from build123d import *

# Parameters (mm, degrees)
BASE_FLANGE1_DEPTH = 20
SKETCH6_R          = 2
CUT_EXTRUDE1_DEPTH = 10
SKETCH7_R          = 2
CUT_EXTRUDE2_DEPTH = 3


# Sheet-metal steps are written as plain solids
with BuildPart() as part:
    # Sketch1 → Base-Flange1 (new body)
    with BuildSketch(Plane(origin=(0, 0, 0), x_dir=(0, 0, -1), z_dir=(1, 0, 0))):
        with BuildLine():
            Line((0, 20), (0, 2))
            ThreePointArc((0, 2), (-0.585786438, 0.585786438), (-2, 0))
            Line((-2, 0), (-20, 0))
            Line((-20, 0), (-20, -3))
            Line((-20, -3), (-2, -3))
            ThreePointArc((-2, -3), (1.535533906, -1.535533906), (3, 2))
            Line((3, 2), (3, 20))
            Line((3, 20), (0, 20))
        make_face()
    extrude(amount=BASE_FLANGE1_DEPTH)

    # Sketch6 → Cut-Extrude1 (cut)
    with BuildSketch(Plane(origin=(0, 0, -3), x_dir=(-1, 0, 0), z_dir=(0, 0, -1))):
        with Locations(Location((-10, 11, 0), (0, 0, 90))):
            Circle(SKETCH6_R)
    extrude(amount=-CUT_EXTRUDE1_DEPTH, mode=Mode.SUBTRACT)

    # Sketch7 → Cut-Extrude2 (cut)
    with BuildSketch(Plane.XZ.offset(3)):
        with Locations(Location((10, 11, 0), (0, 0, 270))):
            Circle(SKETCH7_R)
    extrude(amount=-CUT_EXTRUDE2_DEPTH, mode=Mode.SUBTRACT)


solid = part.part
CAD build for the part. Positions are in the model's coordinates, mm. A direction names the side the tool comes from. Round coordinates to 2 decimals unless told otherwise and drop trailing zeros. Order: outer loops, then holes, each group sorted by start corner. A loop starts at its lowest first (then second) coordinate and runs counter-clockwise, first axis right, second up. Notation, with made-up numbers: (-22, 27) -> (9, 27) arc R18 cw to (9, 53) -> close; hole circle Ø7 at (26, 25.25). An arc over 180 degrees is marked (long way). Write each question's results on one line, items separated by ' | '.
1. Wall check: line 1 along X through (y, z) = (-1.35, 11); line 2 along Z through (x, y) = (10, 16). Give the ranges that are in metal, low to high. Write a range as [from, to].
Findings below:
line 1: x = [0, 8], [12, 20] | line 2: z = [-3, 0]
2. Flat gauge pins, fed straight in: P1, Ø5, axis at x = 10, z = 11, coming from the +Y side; P2, Ø5, axis at x = 10, y = 11, coming from the +Z side; P3, Ø1.5, axis at y = 2, z = 6, coming from the +X side. Where does each tip first touch, or does it go through?
Findings below:
P1: stops at y = 0 | P2: stops at z = 0 | P3: passes through
3. Pull direction Y, two halves, no side cores. Call faces 1 (the face through (0, -1, 4)), 2 (the face through (11.352, 9.526, -1.521)), 3 (the face through (7.6, 0, 10.9)): pulls with the +Y half, pulls with the -Y half, needs draft (parallel to the pull), parting line crosses it, or undercut.
Findings below:
face 1: needs draft | face 2: undercut | face 3: pulls with the +Y half
4. Cut at B-B (x = 10). Give the cut face in (y, z).
Findings below:
outline: (-3, 2) arc R5 ccw to (2, -3) -> (9, -3) -> (9, 0) -> (2, 0) arc R2 cw to (0, 2) -> (0, 9) -> (-3, 9) -> close; (-3, 13) -> (0, 13) -> (0, 20) -> (-3, 20) -> close; (13, -3) -> (20, -3) -> (20, 0) -> (13, 0) -> close
5. Cut at D-D (x = 4.5). Give the cut face in (y, z), plus the area to 3 significant figures.
Findings below:
outline: (-3, 2) arc R5 ccw to (2, -3) -> (20, -3) -> (20, 0) -> (2, 0) arc R2 cw to (0, 2) -> (0, 20) -> (-3, 20) -> close | area: 124 mm²
6. Cut at A-A (z = 11). Give the cut face in (x, y).
Findings below:
outline: (0, -3) -> (8, -3) -> (8, 0) -> (0, 0) -> close; (12, -3) -> (20, -3) -> (20, 0) -> (12, 0) -> close
7. 3-axis set-ups, long thin cutter, end or side, ignore diameter. For faces 4 (the face through (7.6, 11.1, 0)), 5 (the face through (7.6, 10.9, -3)): which of +Z, -Z, +X, -X, +Y, -Y reach the whole face in a straight line?
Findings below:
face 4: +Z, +X, -X, +Y | face 5: -Z, +X, -X, +Y, -Y
